Drawing for the job (mm, zero at the part's lowest x, y, z). Give positions to 0.01 mm unless a question says otherwise; leave off trailing zeros. Write each loop counter-clockwise with the first axis right and the second up, starting at its lowest first coordinate (ties: lowest second). Pieces come first, ordered by that corner, then holes.
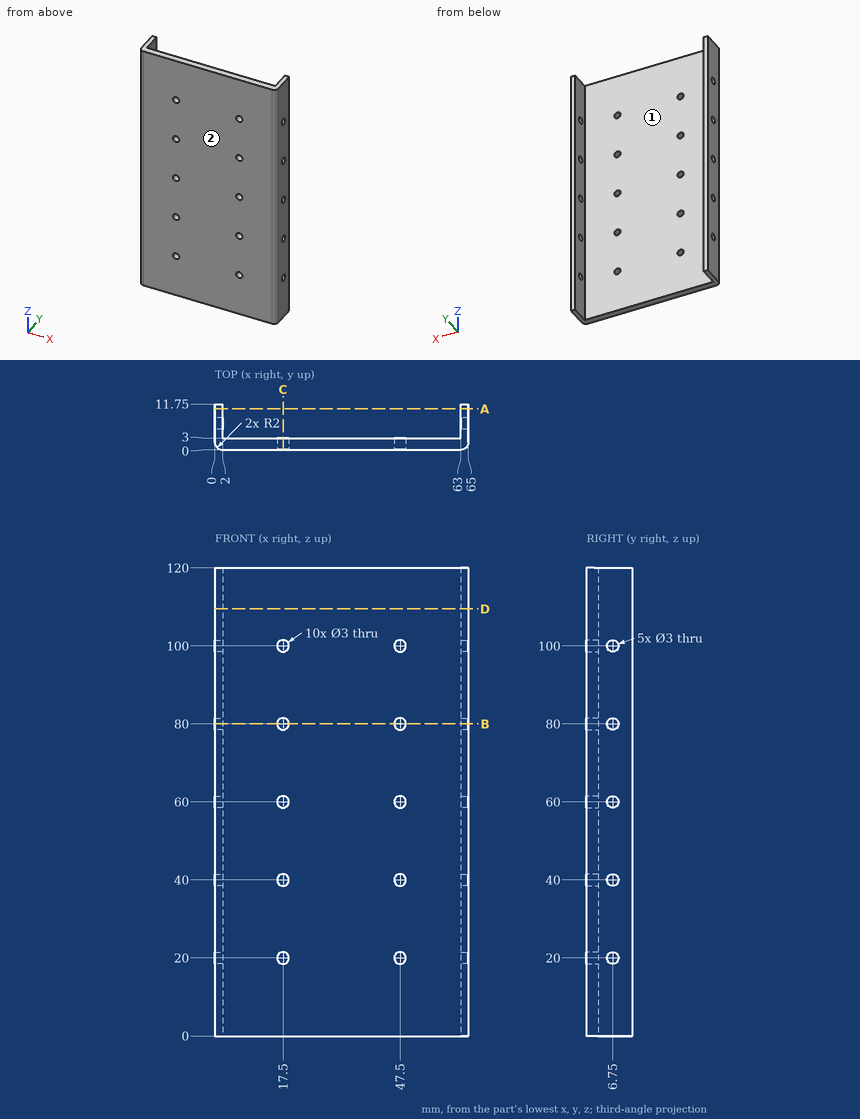
1. Slice it at D-D, the plane z = 109.5. Write the cut outline in (x, y), and give its area (3 significant figures).
Calculated:
outline: (0, 2) arc R2 ccw to (2, 0) - (63, 0) arc R2 ccw to (65, 2) - (65, 11.75) - (63, 11.75) - (63, 3) - (2, 3) - (2, 11.75) - (0, 11.75) - close
area: 228 mm2
2. Pin check, flat tips, straight feed: P1, Ø2.5, axis at x = 17.5, z = 80, coming from the -Y side; P2, Ø5, axis at x = 17.5, z = 20, coming from the +Y side. Stop position of each tip, or through.
Calculated:
P1: passes through
P2: stops at y = 3
3. Slice it at B-B, the plane z = 80. Write the cut outline in (x, y).
Calculated:
outline: (0, 2) arc R2 ccw to (2, 0) - (16, 0) - (16, 3) - (2, 3) - (2, 5.25) - (0, 5.25) - close; (0, 8.25) - (2, 8.25) - (2, 11.75) - (0, 11.75) - close; (19, 0) - (46, 0) - (46, 3) - (19, 3) - close; (49, 0) - (63, 0) arc R2 ccw to (65, 2) - (65, 5.25) - (63, 5.25) - (63, 3) - (49, 3) - close; (63, 8.25) - (65, 8.25) - (65, 11.75) - (63, 11.75) - close
4. Pull direction X, two halves, no side cores. Call the marked faces 1 and 2: +X half, -X half, draft (parallel to the pull), parting line (faces both ways), or undercut.
Calculated:
face 1: undercut
face 2: draft
5. Probe probe 1 along X at (y, z) = (5.5, 41); probe 2 along X at (y, z) = (1.05, 20); probe 3 along Y at (x, z) = (15, 91). List the from-to ranges inside material, lowest first.
Calculated:
probe 1: x = 0 to 2, 63 to 65
probe 2: x = 0.24 to 16, 19 to 46, 49 to 64.76
probe 3: y = 0 to 3
6. Slice it at A-A, the plane y = 10.5. Write the cut outline in (x, z), and give its area (3 significant figures).
Calculated:
outline: (0, 0) - (2, 0) - (2, 120) - (0, 120) - close; (63, 0) - (65, 0) - (65, 120) - (63, 120) - close
area: 480 mm2
7. Slice it at C-C, the plane x = 17.5. Write the cut outline in (y, z), and give its area (3 significant figures).
Calculated:
outline: (0, 0) - (3, 0) - (3, 18.5) - (0, 18.5) - close; (0, 21.5) - (3, 21.5) - (3, 38.5) - (0, 38.5) - close; (0, 41.5) - (3, 41.5) - (3, 58.5) - (0, 58.5) - close; (0, 61.5) - (3, 61.5) - (3, 78.5) - (0, 78.5) - close; (0, 81.5) - (3, 81.5) - (3, 98.5) - (0, 98.5) - close; (0, 101.5) - (3, 101.5) - (3, 120) - (0, 120) - close
area: 315 mm2
